Part model, mm, in its own coordinate system. Face numbers are marked on the shaded views. Coordinates: 2 decimals unless noted, no trailing zeros. Write each loop counter-clockwise with the first axis right and the second up, starting at its lowest first coordinate (ties: lowest second). Pieces come first, ordered by that corner, then holes. Notation, with made-up numbers: (51, 38) - (99, 38) arc R24 cw to (99, 62) - close; hole circle Ø4 at (46.5, 20). An arc over 180 degrees is marked (long way). Write each question's results on one line, items separated by ' | '.
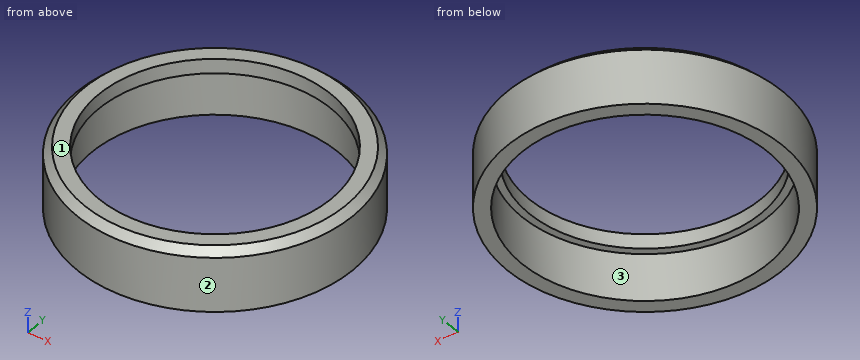
from build123d import *

# Parameters (mm, degrees)
F0_R     = 19
F1_DEPTH = 8.5
F2_R     = 16
F3_DEPTH = 10
F4_R     = 17
F5_DEPTH = 6.5
F6_SIZE  = 1


with BuildPart() as f1:
    # F0 (on Top) → F1 (new body)
    with BuildSketch(Plane.XY):
        Circle(F0_R)
    extrude(amount=F1_DEPTH)

    # F2 (on face) → F3 (cut)
    with BuildSketch(Plane(origin=(0, 0, 0), x_dir=(1, 0, 0), z_dir=(0, 0, -1))):
        Circle(F2_R)
    extrude(amount=-F3_DEPTH, mode=Mode.SUBTRACT)

    # F4 (on face) → F5 (cut)
    with BuildSketch(Plane(origin=(0, 0, 0), x_dir=(1, 0, 0), z_dir=(0, 0, -1))):
        Circle(F4_R)
    extrude(amount=-F5_DEPTH, mode=Mode.SUBTRACT)

    # F6
    f6_edges = [f1.edges().sort_by_distance(p)[0] for p in [
        (-19, 0, 8.5),
    ]]
    chamfer(f6_edges, length=F6_SIZE)


solid = f1.part
(1) Flat gauge pins, fed straight in: P1, Ø1.5, axis at y = 11.5, z = 4.5, coming from the +X side; P2, Ø5, axis at x = 3.5, z = 4.5, coming from the +Y side; P3, Ø5, axis at x = 5, z = 6, coming from the -Y side. Where does each tip first touch, or does it go through?
Return value:
P1: stops at x = 15.67 | P2: stops at y = 18.97 | P3: stops at y = -18.83
(2) Saw through at A-A on y = 0. Write the cut outline in (x, z), then the cut area to 3 significant figures.
Return value:
outline: (-19, 0) - (-17, 0) - (-17, 6.5) - (-16, 6.5) - (-16, 8.5) - (-18, 8.5) - (-19, 7.5) - close; (16, 6.5) - (17, 6.5) - (17, 0) - (19, 0) - (19, 7.5) - (18, 8.5) - (16, 8.5) - close | area: 37.0 mm^2
(3) Saw through at D-D on z = 5.25. Write the cut outline in (x, y).
Return value:
outline: circle Ø38 at (0, 0); hole circle Ø34 at (0, 0)
(4) Saw through at C-C on z = 8. Write the cut outline in (x, y), then the cut area to 3 significant figures.
Return value:
outline: circle Ø37 at (0, 0); hole circle Ø32 at (0, 0) | area: 271 mm^2
(5) Wall check: line 1 (Y direction, x = 0, z = 4.5); line 2 (Y direction, x = 0, z = 7.5); line 3 (X direction, y = -14, z = 5). Give the ranges that are in metal, low to high. Write a range as from..to.
Return value:
line 1: y = -19..-17, 17..19 | line 2: y = -19..-16, 16..19 | line 3: x = -12.85..-9.64, 9.64..12.85
(6) Two-plate mould, pull along X, no slides. Class the marked faces 1, 2 and 3: released by +X, released by -X, zero draft, split by the parting line, or undercut.
Return value:
face 1: zero draft | face 2: split by the parting line | face 3: undercut
